```python
from build123d import *

# Parameters (mm, degrees)
F0_R     = 31.75
F1_DEPTH = 36.83
F2_R     = 25.4
F3_DEPTH = 6.35
F4_SIZE  = 2.54
F5_R     = 19.05
F6_DEPTH = 30.481


with BuildPart() as f1:
    # F0 (on Front) → F1 (new body)
    with BuildSketch(Plane.XZ):
        Circle(F0_R)
    extrude(amount=F1_DEPTH)

    # F2 (on face) → F3 (cut)
    with BuildSketch(Plane.XZ.offset(36.83)):
        Circle(F2_R)
    extrude(amount=-F3_DEPTH, mode=Mode.SUBTRACT)

    # F4
    f4_edges = [f1.edges().sort_by_distance(p)[0] for p in [
        (-25.4, -30.48, 0),
    ]]
    chamfer(f4_edges, length=F4_SIZE)

    # F5 (on face) → F6 (cut, through all)
    with BuildSketch(Plane.XZ.offset(30.48)):
        Circle(F5_R)
    extrude(amount=-F6_DEPTH, mode=Mode.SUBTRACT)


solid = f1.part
```
Check sheet for the modelled part. Datum: model origin and axes. Units: mm. A direction names the side the tool comes from. Round coordinates to 2 decimals unless told otherwise and drop trailing zeros. Order: outer loops, then holes, each group sorted by start corner. A loop starts at its lowest first (then second) coordinate and runs counter-clockwise, first axis right, second up.
1) Scan lines: line 1 (Z direction, x = 0, y = -35); line 2 (Z direction, x = 0, y = -14); line 3 (Y direction, x = 14, z = -13). Record each from-to range of solid material in increasing order.
2) Section check B-B (z = 0). Record the boundary of the cut face in (x, y).
3) Section check A-A (x = 0). Record the boundary of the cut face in (y, z), and give its area (3 significant figures).
4) Go/stop test with flat-tipped pins: pin 1 Ø2 at (x, y) = (-17.5, -21) entering from -Z; pin 2 Ø1 at (x, y) = (24.5, -29) entering from +Z; pin 3 Ø1 at (x, y) = (-1, -15) entering from +Z. Record where each tip stops, or that it passes through.
5) Tool access check on faces 1 (the cylindrical face through (-15.12, -15.45, -11.59)), 2 (the cylindrical face through (-5.506, -34.952, -24.796)). Record the directions out of +Z, -Z, +X, -X, +Y, -Y that give a thin tool (end or side, any length) a straight path to the whole face; none if there is none.
6) Section check C-C (y = -10). Record the boundary of the cut face in (x, z).
7) Mould release check, pull along Z, two halves, no side actions. Record for faces 3 (the flat face through (-14.3, -36.83, 21.3)), 4 (the flat face through (-9, -30.48, 17)), 5 (the cylindrical face through (-6.883, -18.157, -30.995)): +Z half, -Z half, draft (parallel to the pull), parting line (faces both ways), or undercut.
8) Section check D-D (y = -34). Record the boundary of the cut face in (x, z), and give its area (3 significant figures).
Result:
1. line 1: z = -31.75 to -25.4, 25.4 to 31.75
1. line 2: z = -31.75 to -19.05, 19.05 to 31.75
1. line 3: y = -30.48 to 0
2. outline: (-31.75, -36.83) - (-25.4, -36.83) - (-25.4, -33.02) - (-22.86, -30.48) - (-19.05, -30.48) - (-19.05, 0) - (-31.75, 0) - close; (19.05, -30.48) - (22.86, -30.48) - (25.4, -33.02) - (25.4, -36.83) - (31.75, -36.83) - (31.75, 0) - (19.05, 0) - close
3. outline: (-36.83, -31.75) - (0, -31.75) - (0, -19.05) - (-30.48, -19.05) - (-30.48, -22.86) - (-33.02, -25.4) - (-36.83, -25.4) - close; (-36.83, 25.4) - (-33.02, 25.4) - (-30.48, 22.86) - (-30.48, 19.05) - (0, 19.05) - (0, 31.75) - (-36.83, 31.75) - close
3. area: 861 mm2
4. pin 1: stops at z = -27.13
4. pin 2: stops at z = 20.79
4. pin 3: stops at z = 31.75
5. face 1: +Y, -Y
5. face 2: -Y
6. outline: circle Ø63.5 at (0, 0); hole circle Ø38.1 at (0, 0)
7. face 3: draft
7. face 4: undercut
7. face 5: parting line
8. outline: circle Ø63.5 at (0, 0); hole circle Ø50.8 at (0, 0)
8. area: 1,140 mm2
